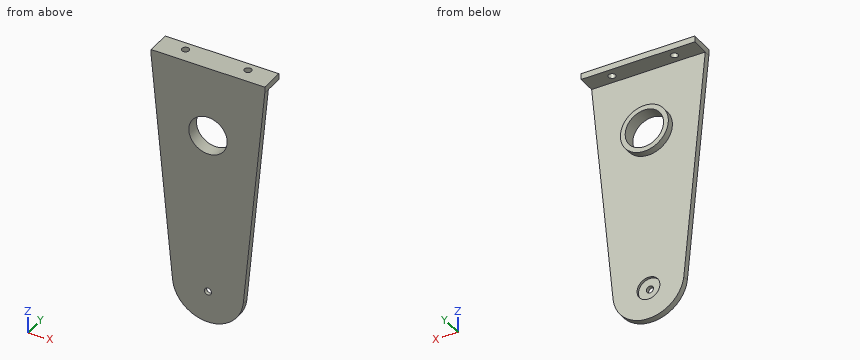
```python
from build123d import *

# Parameters (mm, degrees)
SKETCH2_R           = 1.5
SKETCH2_R_2         = 8
BOSS_EXTRUDE3_DEPTH = 2.54
SKETCH3_W           = 47.380920583
SKETCH3_H           = 10
SKETCH3_R           = 1.5
BOSS_EXTRUDE6_DEPTH = 2.54
SKETCH2_6_R         = 4.7625
SKETCH2_6_R_2       = 1.5
SKETCH2_6_R_3       = 8
SKETCH2_6_R_4       = 6.5
CUT_EXTRUDE2_DEPTH  = 1
SKETCH2_8_R         = 10
SKETCH2_8_R_2       = 8
BOSS_EXTRUDE7_DEPTH = 2.9


with BuildPart() as part:
    # Sketch2 → Boss-Extrude3 (new body)
    with BuildSketch(Plane.XZ):
        with BuildLine():
            Line((14.71851466, 0), (23.68035712, 94.809011723))
            Line((23.68035712, 94.809011723), (-23.700563463, 94.809011723))
            Line((-23.700563463, 94.809011723), (-14.758927346, 0))
            ThreePointArc((-14.758927346, 0), (-0.020206343, -13.282171548), (14.71851466, 0))
        make_face()
        with Locations((-0.020206343, 0)):
            Circle(SKETCH2_R, mode=Mode.SUBTRACT)
        with Locations((-0.000200837, 67.999997057)):
            Circle(SKETCH2_R_2, mode=Mode.SUBTRACT)
    extrude(amount=BOSS_EXTRUDE3_DEPTH)

    # Sketch3 → Boss-Extrude6 (add)
    with BuildSketch(Plane.XY.offset(94.809011723)):
        with Locations((-0.010103172, 2.46)):
            Rectangle(SKETCH3_W, SKETCH3_H)
        with Locations((-13.010103172, 3.73)):
            Circle(SKETCH3_R, mode=Mode.SUBTRACT)
        with Locations((12.989896828, 3.73)):
            Circle(SKETCH3_R, mode=Mode.SUBTRACT)
    extrude(amount=BOSS_EXTRUDE6_DEPTH)

    # Sketch2<6> → Cut-Extrude2 (cut)
    with BuildSketch(Plane.XZ):
        with Locations((-0.020206343, 0)):
            Circle(SKETCH2_6_R)
        with Locations((-0.020206343, 0)):
            Circle(SKETCH2_6_R_2, mode=Mode.SUBTRACT)
        with Locations((-0.000200837, 67.999997057)):
            Circle(SKETCH2_6_R_3)
        with Locations((-0.000200837, 67.999997057)):
            Circle(SKETCH2_6_R_4, mode=Mode.SUBTRACT)
    extrude(amount=CUT_EXTRUDE2_DEPTH, mode=Mode.SUBTRACT)

    # Sketch2<8> → Boss-Extrude7 (add)
    with BuildSketch(Plane.XZ):
        with Locations((-0.000200837, 67.999997057)):
            Circle(SKETCH2_8_R)
        with Locations((-0.000200837, 67.999997057)):
            Circle(SKETCH2_8_R_2, mode=Mode.SUBTRACT)
    extrude(amount=-BOSS_EXTRUDE7_DEPTH)


solid = part.part
```
Source: CAD feature listing. Evaluate the final solid. Frame: model axes, mm. Coordinates: 2 decimals unless noted, no trailing zeros. Write each loop counter-clockwise with the first axis right and the second up, starting at its lowest first coordinate (ties: lowest second). Pieces come first, ordered by that corner, then holes. Notation, with made-up numbers: (9, 51) - (56, 51) arc R20 cw to (56, 58) - close; hole circle Ø10 at (5, 75.25). An arc over 180 degrees is marked (long way). Answer as a JSON object with one key per item and string values.
Q1. Material intervals for line 1 (Y direction, x = -17, z = 28); line 2 (Z direction, x = -18, y = 0.5); line 3 (Z direction, x = 2, y = 2), sorted ascending. Write a range as [from, to].
Ans:
{"line 1": "y = [-2.54, 0]", "line 2": "z = [94.81, 97.35]", "line 3": "z = [58.2, 60.25], [75.75, 77.8], [94.81, 97.35]"}
Q2. First-contact query: pin 1 Ø6 at (x, y) = (-9, 5.5) entering from -Z; pin 2 Ø22 at (x, z) = (-2.5, 68) entering from +Y; pin 3 Ø2.5 at (x, y) = (-13.01, 3.73) entering from +Z; pin 4 Ø4 at (x, y) = (12.99, 3.73) entering from -Z. Flat tips, straight axial feed; report the tip coordinate or a pass-through.
Ans:
{"pin 1": "stops at z = 61.39", "pin 2": "stops at y = 2.9", "pin 3": "passes through", "pin 4": "stops at z = 94.81"}
Q3. Section query D-D, the plane z = 43.5. Output: boundary loops of the cut face in (x, y), plus the area to 3 significant figures.
Ans:
{"outline": "(-18.86, -2.54) - (18.83, -2.54) - (18.83, 0) - (-18.86, 0) - close", "area": "95.7 mm2"}
Q4. Section query C-C, the plane x = 3.5. Output: boundary loops of the cut face in (y, z).
Ans:
{"outline": "(-2.54, -12.86) - (0, -12.86) - (0, -3.21) - (-1, -3.21) - (-1, 3.21) - (0, 3.21) - (0, 58.63) - (2.9, 58.63) - (2.9, 60.81) - (-2.54, 60.81) - close; (-2.54, 75.19) - (2.9, 75.19) - (2.9, 77.37) - (0, 77.37) - (0, 94.81) - (7.46, 94.81) - (7.46, 97.35) - (-2.54, 97.35) - close"}
Q5. Section query B-B, the plane z = 65. Output: boundary loops of the cut face in (x, y), plus the area to 3 significant figures.
Ans:
{"outline": "(-20.89, -2.54) - (-7.42, -2.54) - (-7.42, 2.9) - (-9.54, 2.9) - (-9.54, 0) - (-20.89, 0) - close; (7.42, -2.54) - (20.86, -2.54) - (20.86, 0) - (9.54, 0) - (9.54, 2.9) - (7.42, 2.9) - close", "area": "80.7 mm2"}
Q6. Section query A-A, the plane x = -13. Output: boundary loops of the cut face in (y, z), plus the area to 3 significant figures.
Ans:
{"outline": "(-2.54, -5.61) - (0, -5.61) - (0, 94.81) - (2.23, 94.81) - (2.23, 97.35) - (-2.54, 97.35) - close; (5.23, 94.81) - (7.46, 94.81) - (7.46, 97.35) - (5.23, 97.35) - close", "area": "273 mm2"}
